Check sheet for the drawn part. Datum: minimum x, y, z corner. Units: mm. A direction names the side the tool comes from. Coordinates: 2 decimals unless noted, no trailing zeros. Loops run counter-clockwise (first coordinate to the right, second up) from the corner with the lowest first, then second, coordinate; pieces in that order, holes last. Notation, with made-up numbers: (86, 64) - (142, 64) arc R32 cw to (142, 91) - close; hole circle Ø8 at (-30, 9.5). An arc over 180 degrees is marked (long way). Write item = value, one per line. Start each with the question number.
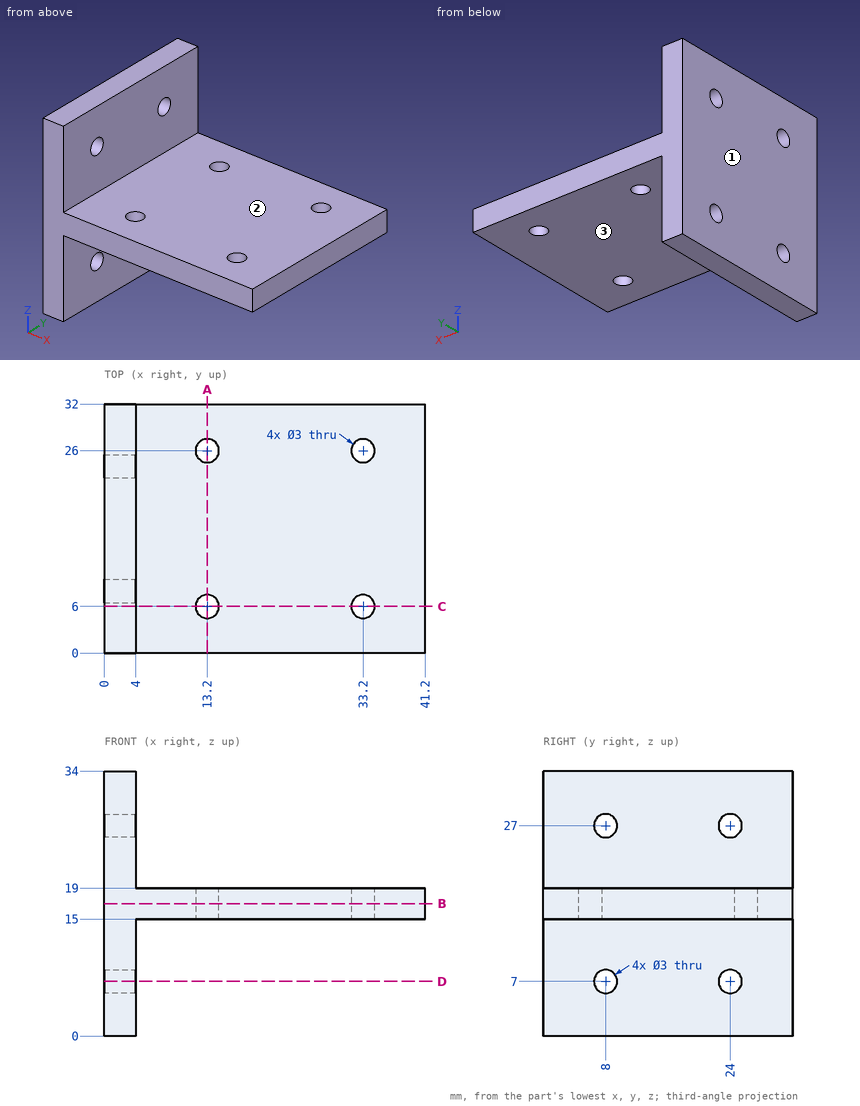
(1) Tool access check on the marked faces 1, 2 and 3. Record the directions out of +Z, -Z, +X, -X, +Y, -Y that give a thin tool (end or side, any length) a straight path to the whole face; none if there is none.
(2) Sectioned sample at D-D on z = 7. Enter the section's corners in (x, y).
(3) Scan lines: line 1 (Y direction, x = 33.2, z = 17.25); line 2 (Y direction, x = 2.8, z = 27); line 3 (X direction, y = 29, z = 25). Record each from-to range of solid material in increasing order.
(4) Sectioned sample at A-A on x = 13.2. Enter the section's corners in (y, z), plus the area to 3 significant figures.
(5) Depth check by flat-ended pin: pin 1 (2.5 mm diameter, centred on y = 24, z = 7, fed in from -X); pin 2 (5 mm diameter, centred on x = 13.2, y = 26, fed in from -Z); pin 3 (16.5 mm diameter, centred on y = 16, z = 30, fed in from +X); pin 4 (1 mm diameter, centred on x = 23, y = 19, fed in from +Z). Enter the tip coordinate at first touch or a pass-through.
(6) Sectioned sample at C-C on y = 6. Enter the section's corners in (x, z), plus the area to 3 significant figures.
(7) Sectioned sample at B-B on z = 17. Enter the section's corners in (x, y), plus the area to 3 significant figures.
Working result:
q1.face_1 = +Z, -Z, -X, +Y, -Y
q1.face_2 = +Z, +X, +Y, -Y
q1.face_3 = -Z, +X, +Y, -Y
q2.outline = (0, 0) - (4, 0) - (4, 6.5) - (0, 6.5) - close; (0, 9.5) - (4, 9.5) - (4, 22.5) - (0, 22.5) - close; (0, 25.5) - (4, 25.5) - (4, 32) - (0, 32) - close
q3.line_1 = 0 to 4.5, 7.5 to 24.5, 27.5 to 32
q3.line_2 = 0 to 6.5, 9.5 to 22.5, 25.5 to 32
q3.line_3 = 0 to 4
q4.outline = (0, 15) - (4.5, 15) - (4.5, 19) - (0, 19) - close; (7.5, 15) - (24.5, 15) - (24.5, 19) - (7.5, 19) - close; (27.5, 15) - (32, 15) - (32, 19) - (27.5, 19) - close
q4.area = 104 mm2
q5.pin_1 = through
q5.pin_2 = 15
q5.pin_3 = 4
q5.pin_4 = 19
q6.outline = (0, 0) - (4, 0) - (4, 15) - (11.7, 15) - (11.7, 19) - (4, 19) - (4, 34) - (0, 34) - close; (14.7, 15) - (31.7, 15) - (31.7, 19) - (14.7, 19) - close; (34.7, 15) - (41.2, 15) - (41.2, 19) - (34.7, 19) - close
q6.area = 261 mm2
q7.outline = (0, 0) - (41.2, 0) - (41.2, 32) - (0, 32) - close; hole circle Ø3 at (13.2, 6); hole circle Ø3 at (13.2, 26); hole circle Ø3 at (33.2, 6); hole circle Ø3 at (33.2, 26)
q7.area = 1,290 mm2
